Work out the finished part from the listing and answer in its coordinate system (mm). Round coordinates to 2 decimals unless told otherwise and drop trailing zeros. Loops run counter-clockwise (first coordinate to the right, second up) from the corner with the lowest first, then second, coordinate; pieces in that order, holes last. Notation, with made-up numbers: M 18.5,89 L 70.5,89 A20 cw 70.5,105 Z; hole C 83,49.25 d10. An arc over 180 degrees is marked long. One line per item, written item: value.
```python
from build123d import *

# Parameters (mm, degrees)
ESBO_O1_R                = 1.25
RESSALTO_EXTRUS_O1_DEPTH = 2
ESBO_O2_R                = 2
CORTE_EXTRUS_O1_DEPTH    = 1


with BuildPart() as part:
    # Esboço1 → Ressalto-extrusão1 (new body)
    with BuildSketch(Plane.XY):
        with BuildLine():
            Line((12.2, 16.7), (-8, 16.7))
            Line((-8, 16.7), (-8, 0.3))
            Line((-8, 0.3), (-1.774823935, 0.3))
            ThreePointArc((-1.774823935, 0.3), (0, -1.8), (1.774823935, 0.3))
            Line((1.774823935, 0.3), (12.2, 0.3))
            Line((12.2, 0.3), (12.2, 16.7))
        make_face()
        Circle(ESBO_O1_R, mode=Mode.SUBTRACT)
        with Locations((0, 14.95)):
            Circle(ESBO_O1_R, mode=Mode.SUBTRACT)
    extrude(amount=RESSALTO_EXTRUS_O1_DEPTH)

    # Esboço2 → Corte-extrusão1 (cut)
    with BuildSketch(Plane.XY.offset(2)):
        with Locations((0, 14.95)):
            Circle(ESBO_O2_R)
        Circle(ESBO_O2_R)
    extrude(amount=-CORTE_EXTRUS_O1_DEPTH, mode=Mode.SUBTRACT)


solid = part.part
```
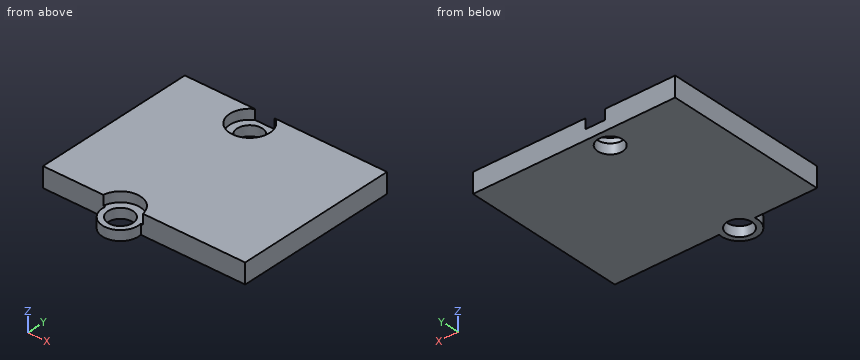
1) Find the intervals of material crossed by probe 1 along Y at (x, z) = (0, 0.25); probe 2 along X at (y, z) = (0, 0.5); probe 3 along X at (y, z) = (14.95, 1.65), in increasing order. Write a range as from..to.
Check values:
probe 1: -1.8..-1.25, 1.25..13.7, 16.2..16.7
probe 2: -1.8..-1.25, 1.25..1.8
probe 3: -8..-2, 2..12.2
2) Find section B-B (x = 0). Give the vertices of the cut face in (y, z), then the cut area to 4 significant figures.
Check values:
outline: M -1.8,0 L -1.25,0 L -1.25,1 L -1.8,1 Z; M 1.25,0 L 13.7,0 L 13.7,1 L 12.95,1 L 12.95,2 L 2,2 L 2,1 L 1.25,1 Z; M 16.2,0 L 16.7,0 L 16.7,1 L 16.2,1 Z
area: 24.45 mm2
3) Find section D-D (y = 14.95). Give the vertices of the cut face in (x, z).
Check values:
outline: M -8,0 L -1.25,0 L -1.25,1 L -2,1 L -2,2 L -8,2 Z; M 1.25,0 L 12.2,0 L 12.2,2 L 2,2 L 2,1 L 1.25,1 Z
4) Find section C-C (z = 0.6). Give the vertices of the cut face in (x, y), then the cut area to 3 significant figures.
Check values:
outline: M -8,0.3 L -1.77,0.3 A1.8 ccw long 1.77,0.3 L 12.2,0.3 L 12.2,16.7 L -8,16.7 Z; hole C 0,0 d2.5; hole C 0,14.95 d2.5
area: 328 mm2
5) Each of these flat-tipped pins is pushed along its axis until it touches: pin 1 (1 mm diameter, centred on x = -4.5, z = 1.5, fed in from -Y); pin 2 (3 mm diameter, centred on x = 0, y = 0, fed in from +Z). Where does it stop, or does it pass through?
Check values:
pin 1: y = 0.3
pin 2: z = 1
6) Find section A-A (y = 0). Give the vertices of the cut face in (x, z).
Check values:
outline: M -1.8,0 L -1.25,0 L -1.25,1 L -1.8,1 Z; M 1.25,0 L 1.8,0 L 1.8,1 L 1.25,1 Z
